Can you work these out from the model? Positions are in its coordinate system, mm. Face numbers are marked on the shaded views. A direction names the side the tool comes from. Coordinates: 2 decimals unless noted, no trailing zeros. Order: outer loops, then holes, each group sorted by start corner. A loop starts at its lowest first (then second) coordinate and runs counter-clockwise, first axis right, second up. Notation, with made-up numbers: (41, 71.25) -> (77, 71.25) arc R4 ccw to (77, 76.25) -> close; hole circle Ø6 at (-27, 74.5). An arc over 180 degrees is marked (long way). Answer as a JSON object with one key per item and string values. Group by question number.
(1) I want a section at B-B, the plane z = 5. List the corners of the cut face in (x, y) for me (3 decimals).
(2) For pin 1 (8.5 mm diameter, centred on y = -17.5, z = 19.5, fed in from -X) (3 decimals); pin 2 (11 mm diameter, centred on y = 28.5, z = 4, fed in from +X) (3 decimals); pin 3 (1.5 mm diameter, centred on y = -26.5, z = 32, fed in from +X); pin 4 (12.5 mm diameter, centred on x = 69.5, y = -9.5, fed in from -Z), each with a flat end and sliding along its axis, tell me the tip position at first contact or that it passes through.
(3) Which directions (+Z, -Z, +X, -X, +Y, -Y) give clear straight access to the entire face, cutting with the end or side of a thin tool? Please do the marked faces 1, 2 and 3.
(4) I need wall thicknesses on line 1 (Z direction, x = 3, y = 13.5) (3 decimals); line 2 (Y direction, x = 5.5, z = 23); line 3 (Y direction, x = 49.5, z = 58). Which ranges of each line are inside material? Lowest first, please.
(5) If we mould it in two halves opening along X, with no side actions, what happens to the marked faces 4, 5, 6 and 7? For each: pulls with the +X half, pulls with the -X half, needs draft (parallel to the pull), parting line crosses it, or undercut.
(6) I want a section at A-A, the plane y = 36. List the corners of the cut face in (x, z) for me (3 decimals), plus the area to 3 significant figures.
from build123d import *

# Parameters (mm, degrees)
F1_DEPTH = 63.5
F2_DEPTH = 25.4
F3_DEPTH = 7.9375


with BuildPart() as f1:
    # F0 (on Front) → F1 (new body, symmetric)
    with BuildSketch(Plane.XZ):
        Polygon((41.275, -9.525), (41.275, 9.525), (22.225, 9.525), (-41.275, 9.525), (-41.275, -9.525), align=None)
    extrude(amount=F1_DEPTH, both=True)

    # F0 (on Front) → F2 (join, symmetric)
    with BuildSketch(Plane.XZ):
        with BuildLine():
            Line((22.225, 9.525), (41.275, 9.525))
            Line((41.275, 9.525), (41.275, 27.00056))
            ThreePointArc((41.275, 27.00056), (45.88692, 38.187993), (57.043019, 42.8752))
            Line((57.043019, 42.8752), (60.325, 42.897318))
            Line((60.325, 42.897318), (60.325, 61.94775))
            Line((60.325, 61.94775), (56.914641, 61.924767))
            add(Edge.make_bspline(
                [(56.039947, 61.907915), (56.331704, 61.913887), (56.623274, 61.919503), (56.914641, 61.924767)],
                knots=[110.599591, 110.599591, 110.599591, 110.599591, 111.296636, 111.296636, 111.296636, 111.296636], degree=3))
            ThreePointArc((56.039947, 61.907915), (32.064903, 51.300633), (22.225, 27.00056))
            Line((22.225, 27.00056), (22.225, 9.525))
        make_face()
        Polygon((60.325, 42.897318), (60.325, 42.8752), (60.325, 38.1), (85.725, 38.1), (85.725, 66.675), (60.325, 66.675), (60.325, 61.94775), align=None)
    extrude(amount=F2_DEPTH, both=True)

    # F0 (on Front) → F3 (join, symmetric)
    with BuildSketch(Plane.XZ):
        with BuildLine():
            Line((-41.275, 9.525), (22.225, 9.525))
            Line((22.225, 9.525), (22.225, 27.00056))
            ThreePointArc((22.225, 27.00056), (32.064903, 51.300633), (56.039947, 61.907915))
            add(Edge.make_bspline(
                [(-41.275, 9.525), (-41.269693, 51.029399), (9.747121, 60.960284), (56.039947, 61.907915)],
                knots=[0, 0, 0, 0, 110.599591, 110.599591, 110.599591, 110.599591], degree=3))
        make_face()
    extrude(amount=F3_DEPTH, both=True)


solid = f1.part
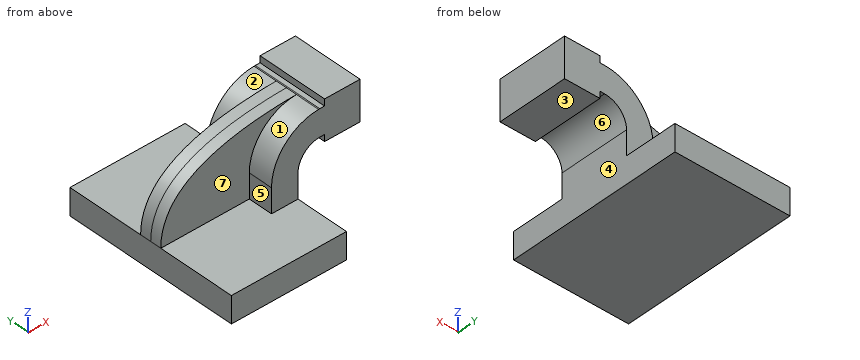
Computed values:
{
 "1": {"outline": "(-41.275, -63.5) -> (41.275, -63.5) -> (41.275, 63.5) -> (-41.275, 63.5) -> close"},
 "2": {"pin 1": "stops at x = 22.225", "pin 2": "stops at x = 41.275", "pin 3": "passes through", "pin 4": "stops at z = 38.1"},
 "3": {"face 1": "+Z, -X, -Y", "face 2": "+Z, -X, +Y", "face 3": "-Z, +X, +Y, -Y"},
 "4": {"line 1": "z = -9.525 to 9.525", "line 2": "y = -7.94 to 7.94", "line 3": "y = -25.4 to 25.4"},
 "5": {"face 4": "pulls with the +X half", "face 5": "pulls with the -X half", "face 6": "undercut", "face 7": "needs draft"},
 "6": {"outline": "(-41.275, -9.525) -> (41.275, -9.525) -> (41.275, 9.525) -> (-41.275, 9.525) -> close", "area": "1,570 mm2"}
}
